Verification items for this drawing (mm, ordinates from the low corner). Give positions to 0.01 mm unless a question says otherwise; leave off trailing zeros. Loops run counter-clockwise (first coordinate to the right, second up) from the corner with the lowest first, then second, coordinate; pieces in that order, holes last. Notation, with made-up numbers: M 5.25,64.5 L 61.25,64.5 A10 ccw 61.25,73.5 Z; hole C 70,64.5 d4. An arc over 180 degrees is marked long. Answer in a Markdown table with one row per item.
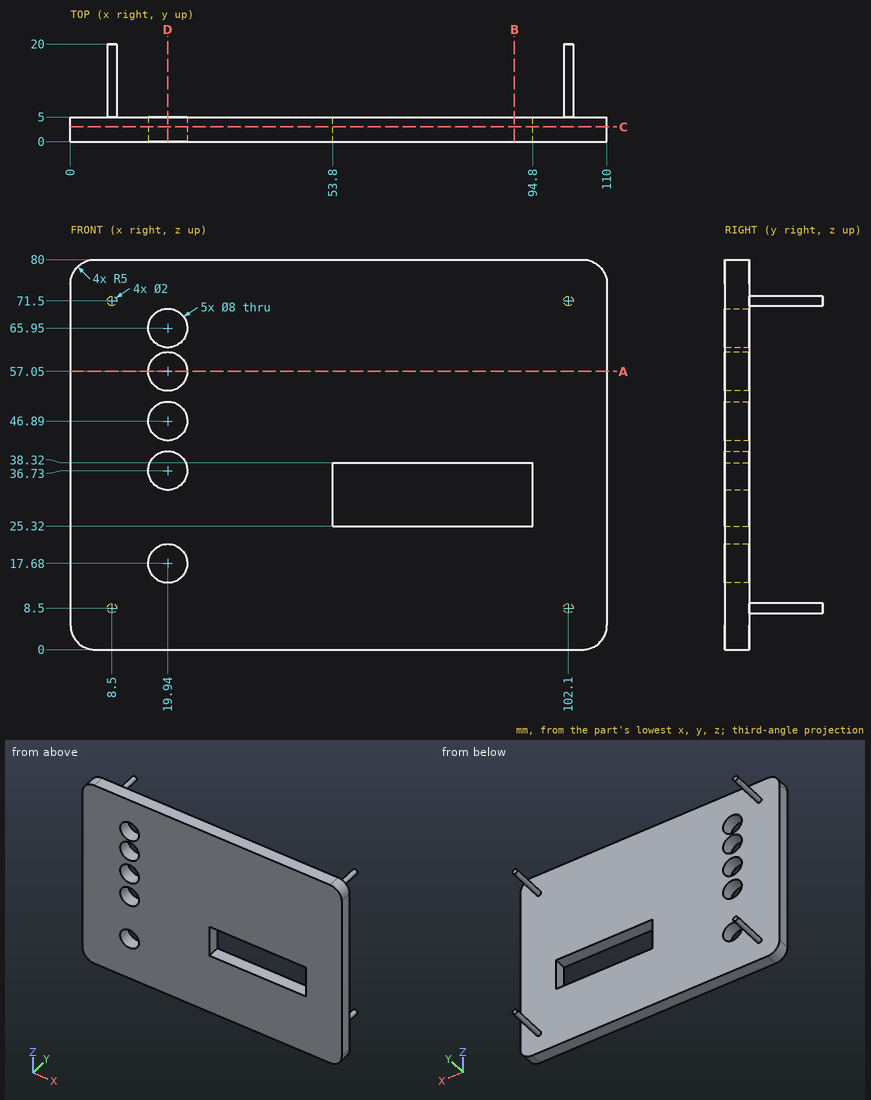
Item 1: Sectioned sample at C-C (y = 3). Record the cut outline in (x, z), and give its area (3 significant figures).
Reported:
| item | result |
|---|---|
| outline | M 0,5 A5 ccw 5,0 L 105,0 A5 ccw 110,5 L 110,75 A5 ccw 105,80 L 5,80 A5 ccw 0,75 Z; hole C 19.94,17.68 d8; hole C 19.94,36.73 d8; hole C 19.94,46.89 d8; hole C 19.94,57.05 d8; hole C 19.94,65.95 d8; hole M 53.8,25.32 L 94.8,25.32 L 94.8,38.32 L 53.8,38.32 Z |
| area | 7,990 mm^2 |
Item 2: Sectioned sample at B-B (x = 91). Record the cut outline in (y, z).
Reported:
| item | result |
|---|---|
| outline | M 0,0 L 5,0 L 5,25.32 L 0,25.32 Z; M 0,38.32 L 5,38.32 L 5,80 L 0,80 Z |
Item 3: Sectioned sample at D-D (x = 19.94). Record the cut outline in (y, z).
Reported:
| item | result |
|---|---|
| outline | M 0,0 L 5,0 L 5,13.68 L 0,13.68 Z; M 0,21.68 L 5,21.68 L 5,32.73 L 0,32.73 Z; M 0,40.73 L 5,40.73 L 5,42.89 L 0,42.89 Z; M 0,50.89 L 5,50.89 L 5,53.05 L 0,53.05 Z; M 0,61.05 L 5,61.05 L 5,61.95 L 0,61.95 Z; M 0,69.95 L 5,69.95 L 5,80 L 0,80 Z |
Item 4: Scan lines: L1, parallel to X at y = 2.3, z = 36.73; L2, parallel to X at y = 2.55, z = 17.68; L3, parallel to Y at x = 87, z = 51. Record each from-to range of solid material in increasing order. Write a range as [from, to].
Reported:
| item | result |
|---|---|
| L1 | x = [0, 15.94], [23.94, 53.8], [94.8, 110] |
| L2 | x = [0, 15.94], [23.94, 110] |
| L3 | y = [0, 5] |
Item 5: Sectioned sample at A-A (z = 57.05). Record the cut outline in (x, y), and give its area (3 significant figures).
Reported:
| item | result |
|---|---|
| outline | M 0,0 L 15.94,0 L 15.94,5 L 0,5 Z; M 23.94,0 L 110,0 L 110,5 L 23.94,5 Z |
| area | 510 mm^2 |
Item 6: Go/stop test with a flat-tipped pin: pin 1 (13 mm diameter, centred on x = 19.94, z = 57.05, fed in from +Y). Record where the tip stops, or that it passes through.
Reported:
| item | result |
|---|---|
| pin 1 | stops at y = 5 |
